from build123d import *

# Parameters (mm, degrees)
SHELL1_T = -2


with BuildPart() as part:
    # Sketch1 → Revolve1 (revolve)
    with BuildSketch(Plane.XY, mode=Mode.PRIVATE) as revolve1_sk:
        with BuildLine():
            Line((0, 0), (60, 0))
            Line((60, 0), (60, 145))
            ThreePointArc((60, 145), (43.890872965, 183.890872965), (5, 200))
            Line((5, 200), (0, 200))
            Line((0, 200), (0, 0))
        make_face()
    revolve(revolve1_sk.sketch.rotate(Axis((0, 200, 0), (0, -1, 0)), 180), axis=Axis((0, 200, 0), (0, -1, 0)))

    # Shell1
    shell1_openings = [part.faces().sort_by_distance(p)[0] for p in [
        (0, 0, 0),
    ]]
    offset(amount=SHELL1_T, openings=shell1_openings, kind=Kind.INTERSECTION)


solid = part.part
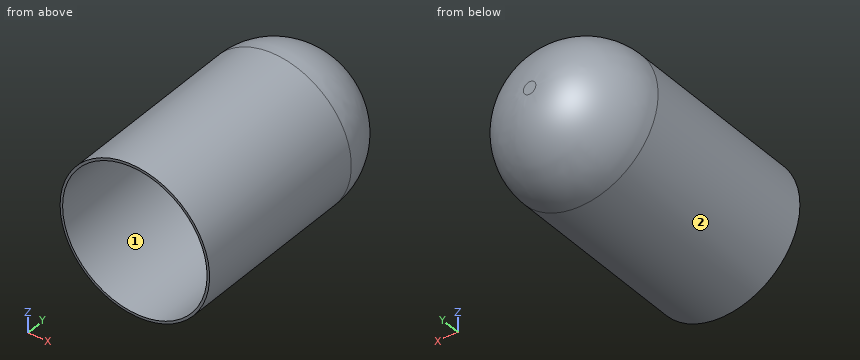
Can you work these out from the model? Positions are in its coordinate system, mm. Face numbers are marked on the shaded views. Round coordinates to 2 decimals unless told otherwise and drop trailing zeros. Loops run counter-clockwise (first coordinate to the right, second up) from the corner with the lowest first, then second, coordinate; pieces in that order, holes last. Notation, with made-up numbers: (77, 7.25) - (102, 7.25) arc R14 cw to (102, 21.25) - close; hole circle Ø7 at (83, 49.5). An arc over 180 degrees is marked (long way). Write item = value, one per line. Start each with the question number.
(1) For P1, Ø10, axis at x = -20.5, y = 49.5, coming from the -Z side; P2, Ø4, axis at x = 47.5, y = 86, coming from the -Z side; P3, Ø12, axis at y = 64, z = -47.5, coming from the +X side, each with a flat end and sliding along its axis, tell me the tip position at first contact or that it passes through.
(2) If I drill on probe 1 along Z at (x, y) = (0, 90); probe 2 along X at (y, z) = (24, -15.5); probe 3 along X at (y, z) = (137, 29), over which ranges is the centre line in solid material (lowest first)? Write a range as [from, to].
(3) If we section it at A-A (y = 123): Please give me the cut outline in (x, z).
(4) If we mould it in two halves opening along Z, with no side actions, what happens to the marked faces 1 and 2? For each: released by +Z, released by -Z, zero draft, split by the parting line, or undercut.
Ans:
q1.P1 = -57.96
q1.P2 = -39.11
q1.P3 = 43.33
q2.probe_1 = [-60, -58], [58, 60]
q2.probe_2 = [-57.96, -55.89], [55.89, 57.96]
q2.probe_3 = [-52.53, -50.23], [50.23, 52.53]
q3.outline = circle Ø120 at (0, 0); hole circle Ø116 at (0, 0)
q4.face_1 = undercut
q4.face_2 = split by the parting line
